from build123d import *

# Parameters (mm, degrees)
SKETCH1_W      = 62
SKETCH1_H      = 23.9
EXTRUDE1_DEPTH = 40
SKETCH2_W      = 20
SKETCH2_H      = 23.9
EXTRUDE2_DEPTH = 30
EXTRUDE3_DEPTH = 75.744916215
SKETCH4_R      = 1.5
EXTRUDE4_DEPTH = 45.763852605
SKETCH5_R      = 3.25
EXTRUDE5_DEPTH = 15.9
SKETCH6_R      = 1.5
EXTRUDE6_DEPTH = 56.966150484


with BuildPart() as part:
    # Sketch1 → Extrude1 (new body)
    with BuildSketch(Plane.XY):
        Rectangle(SKETCH1_W, SKETCH1_H)
    extrude(amount=EXTRUDE1_DEPTH)

    # Sketch2 → Extrude2 (cut)
    with BuildSketch(Plane.XY.offset(40)):
        Rectangle(SKETCH2_W, SKETCH2_H)
    extrude(amount=-EXTRUDE2_DEPTH, mode=Mode.SUBTRACT)

    # Sketch3 → Extrude3 (cut, through all)
    with BuildSketch(Plane(origin=(31, 0, 0), x_dir=(0, 0, -1), z_dir=(1, 0, 0))):
        Polygon((-40, -6.95), (-40, 11.95), (0, 11.95), align=None)
    extrude(amount=-EXTRUDE3_DEPTH, mode=Mode.SUBTRACT)

    # Sketch4 → Extrude4 (cut, through all)
    with BuildSketch(Plane.XY.offset(10)):
        with Locations((-4.95, 2.5875)):
            Circle(SKETCH4_R)
        with Locations((4.95, 2.5875)):
            Circle(SKETCH4_R)
        with Locations((4.95, -7.3125)):
            Circle(SKETCH4_R)
        with Locations((-4.95, -7.3125)):
            Circle(SKETCH4_R)
    extrude(amount=-EXTRUDE4_DEPTH, mode=Mode.SUBTRACT)

    # Sketch5 → Extrude5 (cut)
    with BuildSketch(Plane(origin=(0, 11.95, 0), x_dir=(1, 0, 0), z_dir=(0, 1, 0))):
        with Locations(Location((-16.25, -27, 0), (0, 0, 270))):
            Circle(SKETCH5_R)
        with Locations(Location((-24.75, -27, 0), (0, 0, 270))):
            Circle(SKETCH5_R)
        with Locations(Location((24.75, -27, 0), (0, 0, 270))):
            Circle(SKETCH5_R)
        with Locations(Location((16.25, -27, 0), (0, 0, 270))):
            Circle(SKETCH5_R)
    extrude(amount=-EXTRUDE5_DEPTH, mode=Mode.SUBTRACT)

    # Sketch6 → Extrude6 (cut, through all)
    with BuildSketch(Plane(origin=(0, 11.95, 0), x_dir=(1, 0, 0), z_dir=(0, 1, 0))):
        with Locations(Location((-24.75, -27, 0), (0, 0, 270))):
            Circle(SKETCH6_R)
        with Locations(Location((-16.25, -27, 0), (0, 0, 270))):
            Circle(SKETCH6_R)
        with Locations(Location((16.25, -27, 0), (0, 0, 270))):
            Circle(SKETCH6_R)
        with Locations(Location((24.75, -27, 0), (0, 0, 270))):
            Circle(SKETCH6_R)
    extrude(amount=-EXTRUDE6_DEPTH, mode=Mode.SUBTRACT)


solid = part.part
The listing builds one solid part. Answer for the finished solid, in the listing's coordinates (mm). A direction names the side the tool comes from. Coordinates: 2 decimals unless noted, no trailing zeros. Loops run counter-clockwise (first coordinate to the right, second up) from the corner with the lowest first, then second, coordinate; pieces in that order, holes last. Notation, with made-up numbers: (71, 32) -> (92, 32) arc R30 cw to (92, 59) -> close; hole circle Ø9 at (-15, 28.25). An arc over 180 degrees is marked (long way). Answer in a Markdown table with one row per item. Add a question column.
1. Flat-ended cylindrical pins translate along their axes: P1, Ø2.5, axis at x = 16.25, z = 27, coming from the +Y side; P2, Ø5, axis at x = 19.5, y = -1.5, coming from the +Z side; P3, Ø10, axis at x = 21, z = 25.5, coming from the +Y side; P4, Ø5, axis at x = 4.95, y = -7.31, coming from the -Z side. Find the tip coordinate at first contact, or state that the pin passes through.
2. Consider line 1 (X direction, y = -0.95, z = 27); line 2 (X direction, y = -9.5, z = 23); line 3 (X direction, y = -10, z = 27). Determine where each line is inside the solid, lowest interval first. Write a range as [from, to].
3. The part is cut by section A-A, the plane x = 4.95. Count the separate pieces of the cut face and the enclosed holes in it, then the cut area to 3 significant figures.
4. For faces 3 (the cylindrical face through (25.76, -7.89, 25.89)), 4 (the flat face through (10, -5, 22)), 5 (the flat face through (23, -3.95, 28)), determine the directions among +Z, -Z, +X, -X, +Y, -Y from which every point of the face is accessible in a straight line to the end or side of a thin tool.
5. Determine the mould class of faces 1 (the cylindrical face through (24.893, -2.041, 23.753)), 2 (the flat face through (0, -11.95, 6)) for opening direction X: +X half, -X half, draft (parallel to the pull), parting line (faces both ways), or undercut.
6. The part is cut by section D-D, the plane y = 5.25. Write down the section's boundary in (x, z), then the cut area to 3 significant figures.
7. The part is cut by section B-B, the plane z = 15. Write down the section's boundary in (x, y).
8. The part is cut by section C-C, the plane y = -3. Write down the section's boundary in (x, z).
Answer below:
| question | item | result |
|---|---|---|
| 1 | P1 | through |
| 1 | P2 | z = 33.76 |
| 1 | P3 | y = 2.26 |
| 1 | P4 | z = 0 |
| 2 | line 1 | [-31, -28], [-21.5, -19.5], [-13, -10], [10, 13], [19.5, 21.5], [28, 31] |
| 2 | line 2 | [-31, -10], [10, 31] |
| 2 | line 3 | [-31, -26.25], [-23.25, -17.75], [-14.75, -10], [10, 14.75], [17.75, 23.25], [26.25, 31] |
| 3 | separate pieces | 3 |
| 3 | enclosed holes | 0 |
| 3 | area | 155 mm2 |
| 4 | face 3 | +Y, -Y |
| 4 | face 4 | +Z, +Y, -Y |
| 4 | face 5 | +Y |
| 5 | face 1 | undercut |
| 5 | face 2 | draft |
| 6 | outline | (-31, 0) -> (31, 0) -> (31, 14.18) -> (10, 14.18) -> (10, 10) -> (-10, 10) -> (-10, 14.18) -> (-31, 14.18) -> close |
| 6 | area | 796 mm2 |
| 7 | outline | (-31, -11.95) -> (-10, -11.95) -> (-10, 4.86) -> (-31, 4.86) -> close; (10, -11.95) -> (31, -11.95) -> (31, 4.86) -> (10, 4.86) -> close |
| 8 | outline | (-31, 0) -> (31, 0) -> (31, 31.64) -> (10, 31.64) -> (10, 10) -> (-10, 10) -> (-10, 31.64) -> (-31, 31.64) -> close; hole circle Ø6.5 at (-24.75, 27); hole circle Ø6.5 at (-16.25, 27); hole circle Ø6.5 at (16.25, 27); hole circle Ø6.5 at (24.75, 27) |
